Answer from the drawing. Dimensions are ordinates in mm from the lowest x, y and z of the part. A direction names the side the tool comes from. Give positions to 0.01 mm unless a question says otherwise; leave off trailing zeros. Order: outer loops, then holes, each group sorted by start corner. A loop starts at its lowest first (then second) coordinate and runs counter-clockwise, first axis right, second up.
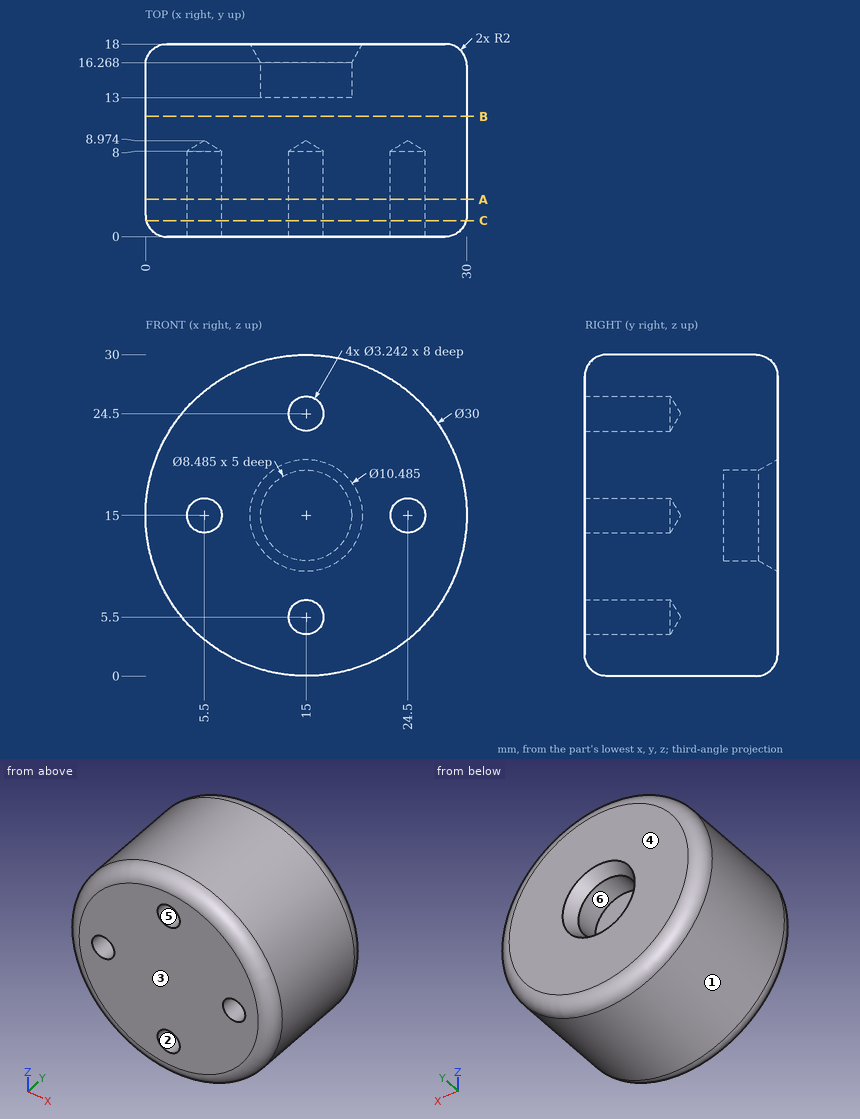
1) The part is cut by section B-B on y = 11.25. Determine the outline of the cut face in (x, z).
Final values:
outline: circle Ø30 at (15, 15)
2) A tool of negligible diameter and unlimited length cuts with its end or side. For the marked faces 4, 5 and 6, from which of +Z, -Z, +X, -X, +Y, -Y can it reach the whole face along a straight path? Write none if from no direction.
Final values:
face 4: +Z, -Z, +X, -X, +Y
face 5: -Y
face 6: +Y
3) For a pull along Z with two mould halves and no side action, classify the marked faces 1, 2 and 3 as released by +Z, released by -Z, zero draft, split by the parting line, or undercut.
Final values:
face 1: split by the parting line
face 2: undercut
face 3: zero draft
4) Given pin 1 (5 mm diameter, centred on y = 6, z = 11.5, fed in from +X); pin 2 (10 mm diameter, centred on x = 18, y = 3, fed in from +Z); pin 3 (4 mm diameter, centred on x = 13.5, z = 16.5, fed in from +Y); pin 4 (1 mm diameter, centred on x = 19, y = 15, fed in from +Z), each flat-ended and moving along its own axis, determine where each tip first touches the part or whether it passes through.
Final values:
pin 1: stops at x = 29.97
pin 2: stops at z = 30
pin 3: stops at y = 13
pin 4: stops at z = 29.59
5) The part is cut by section C-C on y = 1.5. Determine the outline of the cut face in (x, z).
Final values:
outline: circle Ø29.87 at (15, 15); hole circle Ø3.24 at (5.5, 15); hole circle Ø3.24 at (15, 5.5); hole circle Ø3.24 at (15, 24.5); hole circle Ø3.24 at (24.5, 15)
6) The part is cut by section A-A on y = 3.5. Determine the outline of the cut face in (x, z), and give its area (3 significant figures).
Final values:
outline: circle Ø30 at (15, 15); hole circle Ø3.24 at (5.5, 15); hole circle Ø3.24 at (15, 5.5); hole circle Ø3.24 at (15, 24.5); hole circle Ø3.24 at (24.5, 15)
area: 674 mm2
7) Consider L1, parallel to Z at x = 15, y = 6.75; L2, parallel to Z at x = 15, y = 15; L3, parallel to Z at x = 24.5, y = 2. Determine where each line is inside the solid, lowest interval first.
Final values:
L1: z = 0 to 3.88, 7.12 to 22.88, 26.12 to 30
L2: z = 0 to 10.76, 19.24 to 30
L3: z = 3.39 to 13.38, 16.62 to 26.61
